from build123d import *

# Parameters (mm, degrees)
PAD_DEPTH    = 130
SKETCH001_W  = 10
SKETCH001_H  = 130
PAD001_DEPTH = 2.5


with BuildPart() as part:
    # Sketch → Pad (new body)
    with BuildSketch(Plane.XY):
        Polygon((0, 0), (20, 0), (14.505045, 2), (0, 2), align=None)
    extrude(amount=PAD_DEPTH)

    # Sketch001 (on Face1 of Pad) → Pad001 (join)
    with BuildSketch(Plane.XZ):
        with Locations((10, 65)):
            Rectangle(SKETCH001_W, SKETCH001_H)
    extrude(amount=PAD001_DEPTH)


solid = part.part
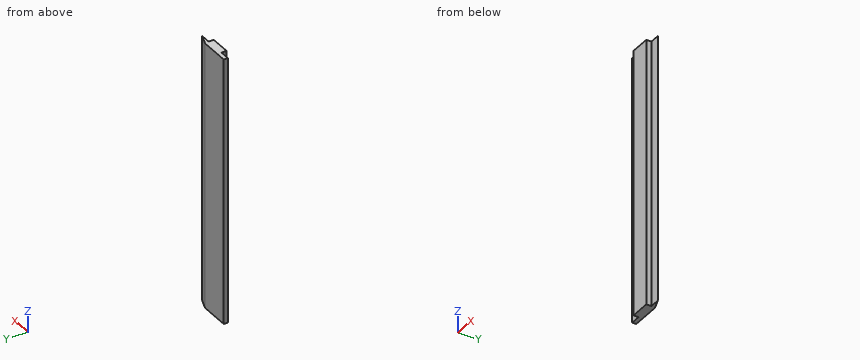
The listing builds one solid part. Answer for the finished solid, in the listing's coordinates (mm). Give positions to 0.01 mm unless a question says otherwise; leave off trailing zeros. Write each loop counter-clockwise with the first axis right and the second up, starting at its lowest first coordinate (ties: lowest second). Pieces come first, ordered by that corner, then holes.
1) Section B-B (x = 3) is taken. Write down the section's boundary in (y, z), and give its area (3 significant figures).
2) Section C-C (y = -0.85) is taken. Write down the section's boundary in (x, z).
3) Find the intervals of material crossed by L1, parallel to X at y = -1.25, z = 74.5; L2, parallel to Y at x = 4.5, z = 60.5; L3, parallel to Y at x = 16.5, z = 33.5, in increasing order.
4) Given P1, Ø2.5, axis at x = 2.5, z = 45.5, coming from the -Y side; P2, Ø1.5, axis at y = -2, z = 51, coming from the +X side, each flat-ended and moving along its own axis, determine where each tip first touches the part or whether it passes through.
5) Section A-A (z = 100) is taken. Write down the section's boundary in (x, y), and give its area (3 significant figures).
Response:
1. outline: (0, 0) - (2, 0) - (2, 130) - (0, 130) - close
1. area: 260 mm2
2. outline: (5, 0) - (15, 0) - (15, 130) - (5, 130) - close
3. L1: x = 5 to 15
3. L2: y = 0 to 2
3. L3: y = 0 to 1.27
4. P1: stops at y = 0
4. P2: stops at x = 15
5. outline: (0, 0) - (5, 0) - (5, -2.5) - (15, -2.5) - (15, 0) - (20, 0) - (14.51, 2) - (0, 2) - close
5. area: 59.5 mm2
